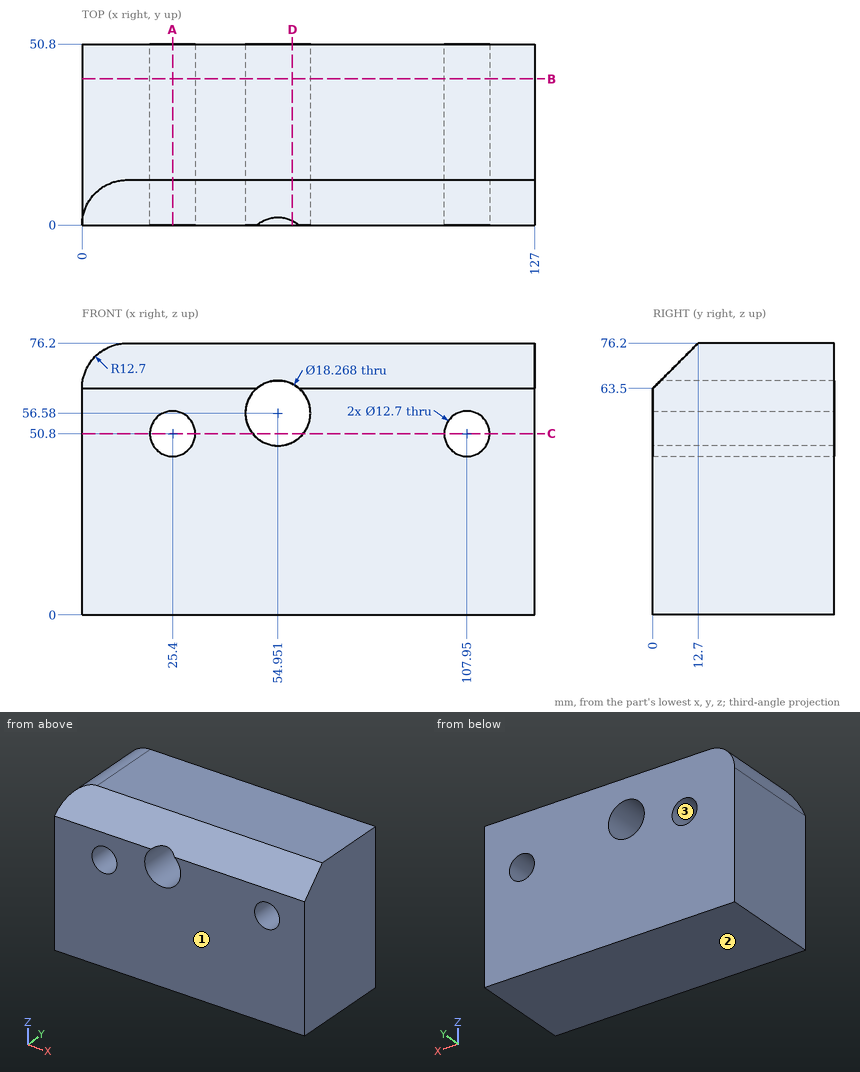
Geometry: see drawing. Coordinates: mm, zero at the bounding-box minimum. Round coordinates to 2 decimals unless told otherwise and drop trailing zeros. Loops run counter-clockwise (first coordinate to the right, second up) from the corner with the lowest first, then second, coordinate; pieces in that order, holes last. Notation, with made-up numbers: (88, 14.25) -> (109, 14.25) arc R22 cw to (109, 21.25) -> close; hole circle Ø7 at (-12, 75). An arc over 180 degrees is marked (long way). Use one line per item in the form item = value. Start each with the question number.
Item 1: Section query B-B on y = 41. Return the cut outline in (x, z) (3 decimals), then the cut area to 3 significant figures.
Item 2: Section query C-C on z = 50.8. Return the cut outline in (x, y), then the cut area to 3 significant figures.
Item 3: Section query D-D on x = 59. Return the cut outline in (y, z).
Item 4: Contact query for a flat-ended pin moving along its axis: pin 1 Ø3 at (y, z) = (18, 66.5) entering from -X. Output: stop coordinate, or through.
Item 5: Section query A-A on x = 25.4. Return the cut outline in (y, z), then the cut area to 3 significant figures.
Item 6: Mould query, pull axis Z, two halves, no side actions, for the marked faces 1, 2 and 3. Classes: pulls with the +Z half, pulls with the -Z half, needs draft (parallel to the pull), parting line crosses it, or undercut.
Item 7: Material intervals for L1, parallel to X at y = 4, z = 49 (1 decimal); L2, parallel to Z at x = 113.5, y = 5 (1 decimal); L3, parallel to X at y = 37, z = 50, sorted ascending. Write a range as from..to.
Ans:
q1.outline = (0, 0) -> (127, 0) -> (127, 76.2) -> (12.7, 76.2) arc R12.7 ccw to (0, 63.5) -> close; hole circle Ø12.7 at (25.4, 50.8); hole circle Ø18.268 at (54.951, 56.58); hole circle Ø12.7 at (107.95, 50.8)
q1.area = 9,130 mm^2
q2.outline = (0, 0) -> (19.05, 0) -> (19.05, 50.8) -> (0, 50.8) -> close; (31.75, 0) -> (47.88, 0) -> (47.88, 50.8) -> (31.75, 50.8) -> close; (62.02, 0) -> (101.6, 0) -> (101.6, 50.8) -> (62.02, 50.8) -> close; (114.3, 0) -> (127, 0) -> (127, 50.8) -> (114.3, 50.8) -> close
q2.area = 4,440 mm^2
q3.outline = (0, 0) -> (50.8, 0) -> (50.8, 48.39) -> (0, 48.39) -> close; (1.27, 64.77) -> (50.8, 64.77) -> (50.8, 76.2) -> (12.7, 76.2) -> close
q4.pin_1 = 0.09
q5.outline = (0, 0) -> (50.8, 0) -> (50.8, 44.45) -> (0, 44.45) -> close; (0, 57.15) -> (50.8, 57.15) -> (50.8, 76.2) -> (12.7, 76.2) -> (0, 63.5) -> close
q5.area = 3,150 mm^2
q6.face_1 = needs draft
q6.face_2 = pulls with the -Z half
q6.face_3 = undercut
q7.L1 = 0..19.3, 31.5..49.9, 60..101.9, 114..127
q7.L2 = 0..47.7, 53.9..68.5
q7.L3 = 0..19.1, 31.7..48.62, 61.29..101.65, 114.25..127
